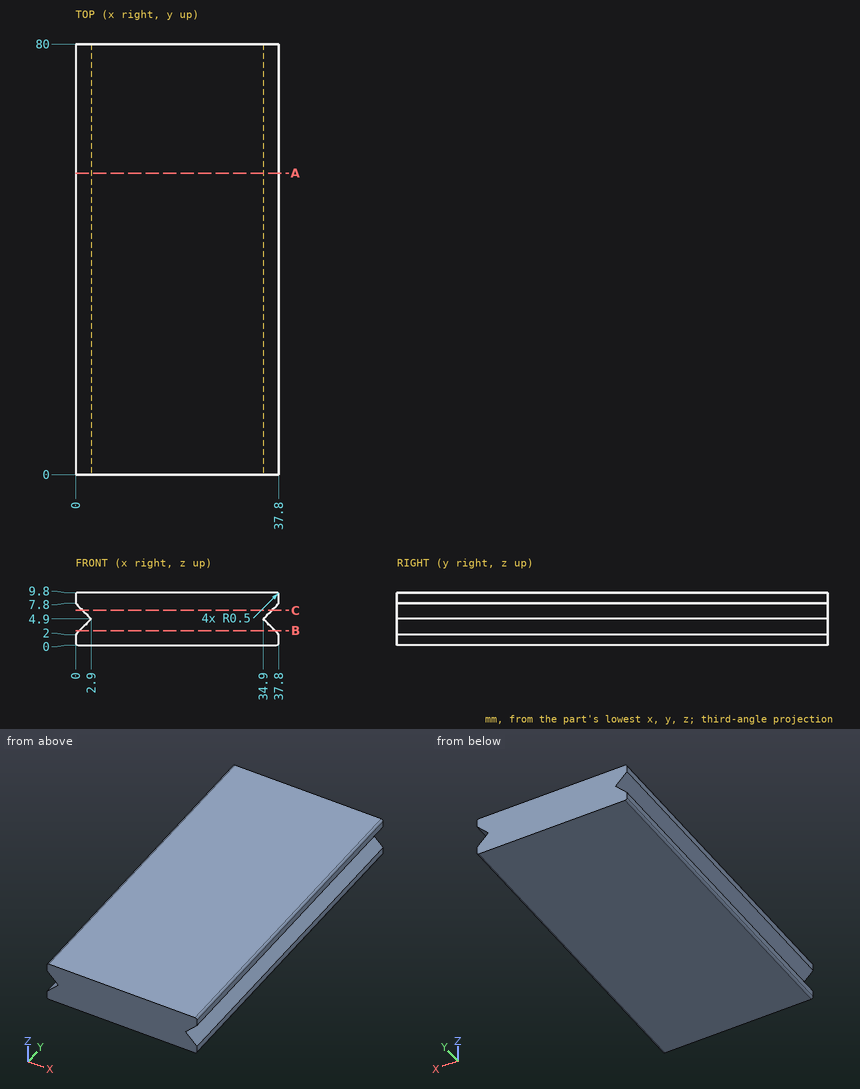
Design review of the part shown in the three views and the two pictorial views. Dimensions are in mm from the part's minimum x, y and z. Coordinates: 2 decimals unless noted, no trailing zeros. Order: outer loops, then holes, each group sorted by start corner. A loop starts at its lowest first (then second) coordinate and runs counter-clockwise, first axis right, second up.
Item 1: Take a section at B-B, the plane z = 2.75. Write out the cut boundary in (x, y).
Item 2: For pin 1 Ø1 at (x, y) = (31.5, 70) entering from -Z, flat-tipped, find the tip position at first contact; note if it passes through.
Item 3: Take a section at C-C, the plane z = 6.5. Write out the cut boundary in (x, y), then the cut area to 3 significant figures.
Item 4: For line 1 (X direction, y = 28.5, z = 2.5); line 2 (X direction, y = 48.5, z = 3), list the stretches that pass through material, from the lowest coordinate up.
Item 5: Take a section at A-A, the plane y = 56. Write out the cut boundary in (x, z), then the cut area to 3 significant figures.
The answers:
1. outline: (0.75, 0) - (37.05, 0) - (37.05, 80) - (0.75, 80) - close
2. pin 1: stops at z = 0
3. outline: (1.3, 0) - (36.5, 0) - (36.5, 80) - (1.3, 80) - close
3. area: 2,820 mm2
4. line 1: x = 0.5 to 37.3
4. line 2: x = 1 to 36.8
5. outline: (0, 0.5) arc R0.5 ccw to (0.5, 0) - (37.3, 0) arc R0.5 ccw to (37.8, 0.5) - (37.8, 2) - (34.9, 4.9) - (37.8, 7.8) - (37.8, 9.3) arc R0.5 ccw to (37.3, 9.8) - (0.5, 9.8) arc R0.5 ccw to (0, 9.3) - (0, 7.8) - (2.9, 4.9) - (0, 2) - close
5. area: 353 mm2
